from build123d import *

# Parameters (mm, degrees)
BOSS_EXTRUDE1_DEPTH     = 13
SKETCH6_W               = 6
SKETCH6_H               = 5
BOSS_EXTRUDE4_DEPTH     = 5.6
SKETCH16_W              = 6
SKETCH16_H              = 8
BOSS_EXTRUDE5_DEPTH     = 0.1
CUT_EXTRUDE6_DEPTH      = 4
CUT_EXTRUDE6_DEPTH_BACK = 3.6
SKETCH15_R              = 1.3
CUT_EXTRUDE7_DEPTH      = 8.7202
CUT_EXTRUDE8_START      = -0.2202
SKETCH19_W              = 6
SKETCH19_H              = 8
SKETCH19_R              = 1.3
CUT_EXTRUDE8_DEPTH      = 0.2202
SKETCH12_R              = 1.5
CUT_EXTRUDE5_DEPTH      = 6
CHAMFER1_SIZE           = 0.2
SKETCH20_W              = 5
SKETCH20_H              = 5.5
BOSS_EXTRUDE6_DEPTH     = 0.5
SKETCH21_W              = 5
SKETCH21_H              = 5.5
BOSS_EXTRUDE7_DEPTH     = 0.5
CHAMFER2_SIZE           = 0.2
CROQUIS1_W              = 5
CROQUIS1_H              = 5.5
CORTAR_EXTRUIR1_DEPTH   = 0.5


with BuildPart() as part:
    # Sketch1 → Boss-Extrude1 (new body)
    with BuildSketch(Plane.XY):
        Polygon((3, 3.05), (3, -2.253801214), (2.388188946, -2.95), (-2.388188946, -2.95), (-3, -2.253801214), (-3, 3.05), align=None)
    extrude(amount=BOSS_EXTRUDE1_DEPTH)

    # Sketch6 → Boss-Extrude4 (add)
    with BuildSketch(Plane(origin=(0, 3.05, 0), x_dir=(1, 0, 0), z_dir=(0, 1, 0))):
        with Locations((0, -2.5)):
            Rectangle(SKETCH6_W, SKETCH6_H)
    extrude(amount=BOSS_EXTRUDE4_DEPTH)

    # Sketch16 → Boss-Extrude5 (add)
    with BuildSketch(Plane(origin=(0, 3.05, 0), x_dir=(1, 0, 0), z_dir=(0, 1, 0))):
        with Locations((0, -9)):
            Rectangle(SKETCH16_W, SKETCH16_H)
    extrude(amount=BOSS_EXTRUDE5_DEPTH)

    # Sketch18 → Cut-Extrude6 (cut, two sides: drawn at the far end of the back side and taken through both)
    with BuildSketch(Plane(origin=(0, 0, 0), x_dir=(0, 0, -1), z_dir=(1, 0, 0)).offset(-CUT_EXTRUDE6_DEPTH_BACK)):
        with BuildLine():
            Line((-8.8572, -0.0702), (-12.8572, -0.0702))
            Line((-12.8572, -0.0702), (-13, -0.0702))
            Line((-13, -0.0702), (-13, -0.7))
            Line((-13, -0.7), (-12.8572, -0.7))
            Line((-12.8572, -0.7), (-12.7144, -0.7))
            add(Edge.make_bspline(
                [(-12.7144, -0.7), (-12.5198, -0.7), (-12.43, -0.9509)],
                knots=[0.103448276, 0.103448276, 0.103448276, 0.137931034, 0.137931034, 0.137931034], degree=2))
            add(Edge.make_bspline(
                [(-12.43, -0.9509), (-12.3594, -1.2388), (-12.13, -1.45), (-11.8572, -1.45)],
                knots=[0.137931034, 0.137931034, 0.137931034, 0.137931034, 0.172413793, 0.172413793, 0.172413793, 0.172413793], degree=3))
            add(Edge.make_bspline(
                [(-11.8572, -1.45), (-11.5844, -1.45), (-11.355, -1.2388), (-11.2844, -0.9509)],
                knots=[0.172413793, 0.172413793, 0.172413793, 0.172413793, 0.206896552, 0.206896552, 0.206896552, 0.206896552], degree=3))
            add(Edge.make_bspline(
                [(-11.2844, -0.9509), (-11.1946, -0.7), (-11, -0.7)],
                knots=[0.206896552, 0.206896552, 0.206896552, 0.24137931, 0.24137931, 0.24137931], degree=2))
            Line((-11, -0.7), (-10.8572, -0.7))
            Line((-10.8572, -0.7), (-10.7144, -0.7))
            add(Edge.make_bspline(
                [(-10.7144, -0.7), (-10.5198, -0.7), (-10.43, -0.9509)],
                knots=[0.310344828, 0.310344828, 0.310344828, 0.344827586, 0.344827586, 0.344827586], degree=2))
            add(Edge.make_bspline(
                [(-10.43, -0.9509), (-10.3594, -1.2388), (-10.13, -1.45), (-9.8572, -1.45)],
                knots=[0.344827586, 0.344827586, 0.344827586, 0.344827586, 0.379310345, 0.379310345, 0.379310345, 0.379310345], degree=3))
            add(Edge.make_bspline(
                [(-9.8572, -1.45), (-9.5844, -1.45), (-9.355, -1.2388), (-9.2844, -0.9509)],
                knots=[0.379310345, 0.379310345, 0.379310345, 0.379310345, 0.413793103, 0.413793103, 0.413793103, 0.413793103], degree=3))
            add(Edge.make_bspline(
                [(-9.2844, -0.9509), (-9.1946, -0.7), (-9, -0.7)],
                knots=[0.413793103, 0.413793103, 0.413793103, 0.448275862, 0.448275862, 0.448275862], degree=2))
            Line((-9, -0.7), (-8.8572, -0.7))
            Line((-8.8572, -0.7), (-8.7144, -0.7))
            add(Edge.make_bspline(
                [(-8.7144, -0.7), (-8.5198, -0.7), (-8.43, -0.9509)],
                knots=[0.517241379, 0.517241379, 0.517241379, 0.551724138, 0.551724138, 0.551724138], degree=2))
            add(Edge.make_bspline(
                [(-8.43, -0.9509), (-8.3594, -1.2388), (-8.13, -1.45), (-7.8572, -1.45)],
                knots=[0.551724138, 0.551724138, 0.551724138, 0.551724138, 0.586206897, 0.586206897, 0.586206897, 0.586206897], degree=3))
            add(Edge.make_bspline(
                [(-7.8572, -1.45), (-7.5844, -1.45), (-7.355, -1.2388), (-7.2844, -0.9509)],
                knots=[0.586206897, 0.586206897, 0.586206897, 0.586206897, 0.620689655, 0.620689655, 0.620689655, 0.620689655], degree=3))
            add(Edge.make_bspline(
                [(-7.2844, -0.9509), (-7.1946, -0.7), (-7, -0.7)],
                knots=[0.620689655, 0.620689655, 0.620689655, 0.655172414, 0.655172414, 0.655172414], degree=2))
            Line((-7, -0.7), (-6.8572, -0.7))
            Line((-6.8572, -0.7), (-6.7144, -0.7))
            add(Edge.make_bspline(
                [(-6.7144, -0.7), (-6.5198, -0.7), (-6.43, -0.9509)],
                knots=[0.724137931, 0.724137931, 0.724137931, 0.75862069, 0.75862069, 0.75862069], degree=2))
            add(Edge.make_bspline(
                [(-6.43, -0.9509), (-6.3594, -1.2388), (-6.13, -1.45), (-5.8572, -1.45)],
                knots=[0.75862069, 0.75862069, 0.75862069, 0.75862069, 0.793103448, 0.793103448, 0.793103448, 0.793103448], degree=3))
            add(Edge.make_bspline(
                [(-5.8572, -1.45), (-5.5844, -1.45), (-5.355, -1.2388), (-5.2844, -0.9509)],
                knots=[0.793103448, 0.793103448, 0.793103448, 0.793103448, 0.827586207, 0.827586207, 0.827586207, 0.827586207], degree=3))
            add(Edge.make_bspline(
                [(-5.2844, -0.9509), (-5.1946, -0.7), (-5, -0.7)],
                knots=[0.827586207, 0.827586207, 0.827586207, 0.862068966, 0.862068966, 0.862068966], degree=2))
            Line((-5, -0.7), (-5, -0.0702))
            Line((-5, -0.0702), (-8.8572, -0.0702))
        make_face()
    extrude(amount=CUT_EXTRUDE6_DEPTH + CUT_EXTRUDE6_DEPTH_BACK, mode=Mode.SUBTRACT)

    # Sketch15 → Cut-Extrude7 (cut)
    with BuildSketch(Plane(origin=(0, 8.65, 0), x_dir=(1, 0, 0), z_dir=(0, 1, 0))):
        with Locations(Location((0, -10.8572, 0), (0, 0, 180))):
            Circle(SKETCH15_R)
        with Locations(Location((0, -6.8572, 0), (0, 0, 180))):
            Circle(SKETCH15_R)
    extrude(amount=-CUT_EXTRUDE7_DEPTH, mode=Mode.SUBTRACT)

    # Sketch19 → Cut-Extrude8 (cut)
    with BuildSketch(Plane.XZ.offset(0.0702).offset(CUT_EXTRUDE8_START)):
        with Locations((0, 9)):
            Rectangle(SKETCH19_W, SKETCH19_H)
        with Locations(Location((0, 10.8572, 0), (0, 0, 180))):
            Circle(SKETCH19_R, mode=Mode.SUBTRACT)
        with Locations(Location((0, 6.8572, 0), (0, 0, 180))):
            Circle(SKETCH19_R, mode=Mode.SUBTRACT)
    extrude(amount=CUT_EXTRUDE8_DEPTH, mode=Mode.SUBTRACT)

    # Sketch12 → Cut-Extrude5 (cut)
    with BuildSketch(Plane.XY.offset(5)):
        with Locations((0, 5.9)):
            Circle(SKETCH12_R)
    extrude(amount=-CUT_EXTRUDE5_DEPTH, mode=Mode.SUBTRACT)

    # Chamfer1
    chamfer1_edges = [part.edges().sort_by_distance(p)[0] for p in [
        (-2.694094473, -2.601900607, 13),
        (0, -2.95, 13),
        (2.694094473, -2.601900607, 13),
        (3, 1.65, 13),
        (3, -1.476900607, 13),
        (-3, -1.476900607, 13),
        (-3, 1.65, 13),
    ]]
    chamfer(chamfer1_edges, length=CHAMFER1_SIZE)

    # Sketch20 → Boss-Extrude6 (add)
    with BuildSketch(Plane(origin=(3, 0, 0), x_dir=(0, 0, -1), z_dir=(1, 0, 0))):
        with Locations((-2.5, 5.9)):
            Rectangle(SKETCH20_W, SKETCH20_H)
    extrude(amount=BOSS_EXTRUDE6_DEPTH)

    # Sketch21 → Boss-Extrude7 (add)
    with BuildSketch(Plane.ZY.offset(3)):
        with Locations((2.5, 5.9)):
            Rectangle(SKETCH21_W, SKETCH21_H)
    extrude(amount=BOSS_EXTRUDE7_DEPTH)

    # Chamfer2
    chamfer2_edges = [part.edges().sort_by_distance(p)[0] for p in [
        (3.5, 5.9, 5),
        (-3.5, 5.9, 5),
    ]]
    chamfer(chamfer2_edges, length=CHAMFER2_SIZE)

    # Croquis1 → Cortar-Extruir1 (cut)
    with BuildSketch(Plane.ZY.offset(3.5)):
        with Locations((2.5, 5.9)):
            Rectangle(CROQUIS1_W, CROQUIS1_H)
    extrude(amount=-CORTAR_EXTRUIR1_DEPTH, mode=Mode.SUBTRACT)


solid = part.part
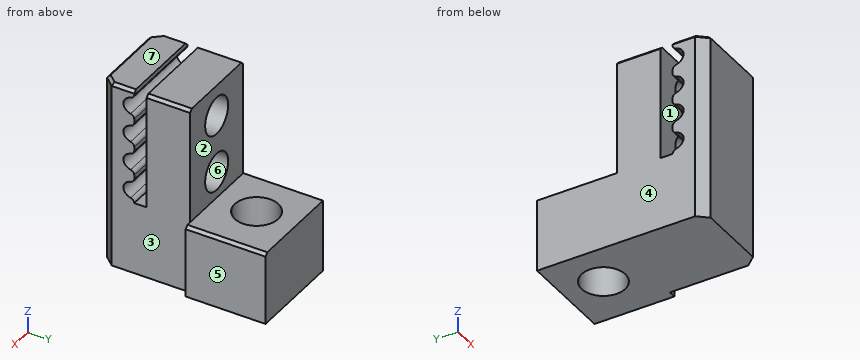
The listing builds one solid part. Answer for the finished solid, in the listing's coordinates (mm). Face numbers are marked on the shaded views. A direction names the side the tool comes from. Coordinates: 2 decimals unless noted, no trailing zeros. Loops run counter-clockwise (first coordinate to the right, second up) from the corner with the lowest first, then second, coordinate; pieces in that order, holes last. Notation, with made-up numbers: (40.5, 78) -> (79.5, 78) arc R16 cw to (79.5, 94) -> close; hole circle Ø10 at (74, -14.5). An arc over 180 degrees is marked (long way). Answer in a Markdown table with one row per item. Add a question column.
1. The part is cut by section B-B, the plane z = 2.5. Write down the section's boundary in (x, y).
2. The part is cut by section C-C, the plane x = 0. Count the separate pieces of the cut face and the enclosed holes in it, then the cut area to 3 significant figures.
3. For the marked faces 1, 2 and 3, determine the directions among +Z, -Z, +X, -X, +Y, -Y from which every point of the face is accessible in a straight line to the end or side of a thin tool.
4. The part is cut by section A-A, the plane y = 5.9. Write down the section's boundary in (x, z).
5. Flat-ended cylindrical pins translate along their axes: P1, Ø2.5, axis at y = 0.5, z = 7.5, coming from the +X side; P2, Ø1.8, axis at x = -0.5, z = 9.5, coming from the +Y side. Find the tip coordinate at first contact, or state that the pin passes through.
6. Consider line 1 (Z direction, x = 0, y = 1.9); line 2 (Z direction, x = 1, y = 3.5); line 3 (Y direction, x = -1.75, z = 8). Determine where each line is inside the solid, lowest interval first. Write a range as [from, to].
7. The part is cut by section D-D, the plane y = 7.25. Write down the section's boundary in (x, z), then the cut area to 3 significant figures.
8. Determine the mould class of the marked faces 4, 5, 6 and 7 for opening direction X: +X half, -X half, draft (parallel to the pull), parting line (faces both ways), or undercut.
Answer below:
| question | item | result |
|---|---|---|
| 1 | outline | (-3, -2.25) -> (-2.39, -2.95) -> (2.39, -2.95) -> (3, -2.25) -> (3, 3.15) -> (3.5, 3.15) -> (3.5, 8.65) -> (-3, 8.65) -> close; hole circle Ø3 at (0, 5.9) |
| 2 | separate pieces | 4 |
| 2 | enclosed holes | 0 |
| 2 | area | 66.4 mm2 |
| 3 | face 1 | +Z, +X, -X |
| 3 | face 2 | +Z, +X, -X, +Y |
| 3 | face 3 | +Z, -Z, +X, -Y |
| 4 | outline | (-3, 0) -> (-1.5, 0) -> (-1.5, 5) -> (-3, 5) -> close; (1.5, 0) -> (3.5, 0) -> (3.5, 4.8) -> (3.3, 5) -> (1.5, 5) -> close |
| 5 | P1 | x = 3 |
| 5 | P2 | y = 3.15 |
| 6 | line 1 | [0, 5.56], [8.16, 9.56], [12.16, 13] |
| 6 | line 2 | [0, 5] |
| 6 | line 3 | [-2.95, -1.43], [0.15, 3.15] |
| 7 | outline | (-3, 0) -> (-0.65, 0) -> (-0.65, 5) -> (-3, 5) -> close; (0.65, 0) -> (3.5, 0) -> (3.5, 4.8) -> (3.3, 5) -> (0.65, 5) -> close |
| 7 | area | 25.9 mm2 |
| 8 | face 4 | -X half |
| 8 | face 5 | +X half |
| 8 | face 6 | undercut |
| 8 | face 7 | draft |
